Geometry check sheet. Reference: drawing and pictorial views, mm from the part's lowest x, y, z. A direction names the side the tool comes from. Coordinates: 2 decimals unless noted, no trailing zeros. Write each loop counter-clockwise with the first axis right and the second up, starting at its lowest first coordinate (ties: lowest second). Pieces come first, ordered by that corner, then holes. Notation, with made-up numbers: (-26, 18) -> (29, 18) arc R4 cw to (29, 24) -> close; hole circle Ø9 at (-16.5, -38.5). An arc over 180 degrees is marked (long way). Use a Markdown table: item, result.
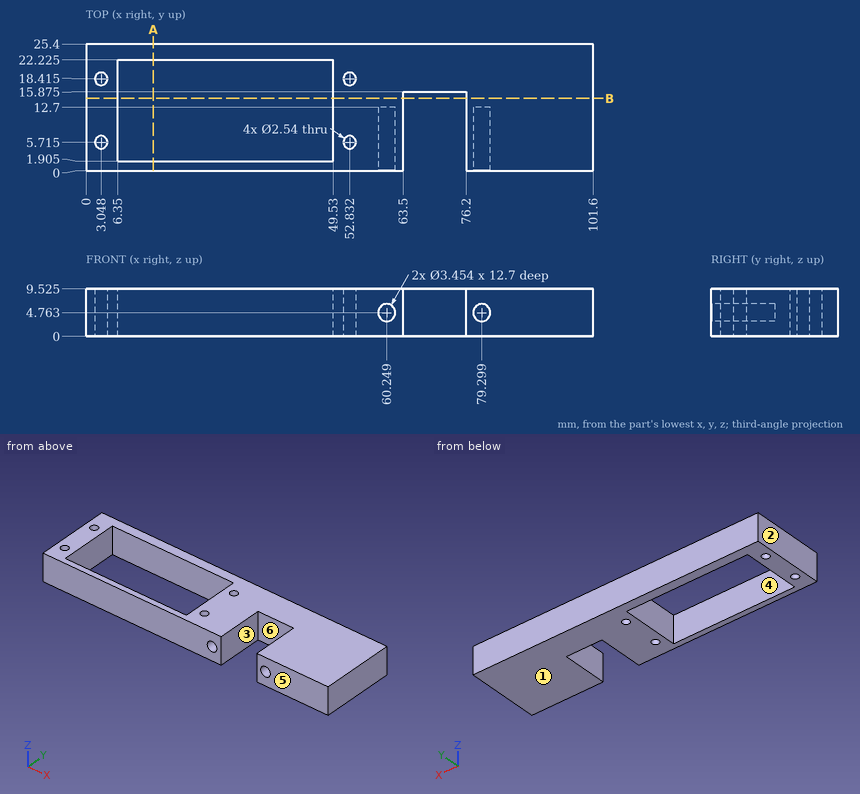
Item 1: Thickness scan on L1, parallel to Y at x = 46, z = 9.25 (1 decimal); L2, parallel to X at y = 3, z = 7.5; L3, parallel to X at y = 20.25, z = 1.75. Record the ranges inside material, lowest first. Write a range as [from, to].
Answer block:
| item | result |
|---|---|
| L1 | y = [0, 1.9], [22.2, 25.4] |
| L2 | x = [0, 6.35], [49.53, 63.5], [76.2, 101.6] |
| L3 | x = [0, 6.35], [49.53, 101.6] |
Item 2: Section check A-A on x = 13.5. Record the boundary of the cut face in (y, z) (1 decimal).
Answer block:
| item | result |
|---|---|
| outline | (0, 0) -> (1.9, 0) -> (1.9, 9.5) -> (0, 9.5) -> close; (22.2, 0) -> (25.4, 0) -> (25.4, 9.5) -> (22.2, 9.5) -> close |
Item 3: Section check B-B on y = 14.5. Count the separate pieces of the cut face and the enclosed holes in it.
Answer block:
| item | result |
|---|---|
| separate pieces | 3 |
| enclosed holes | 0 |
Item 4: Mould release check, pull along X, two halves, no side actions. Record for the marked faces 1, 2 and 3: +X half, -X half, draft (parallel to the pull), parting line (faces both ways), or undercut.
Answer block:
| item | result |
|---|---|
| face 1 | draft |
| face 2 | -X half |
| face 3 | undercut |
Item 5: Tool access check on the marked faces 4, 5 and 6. Record the directions out of +Z, -Z, +X, -X, +Y, -Y that give a thin tool (end or side, any length) a straight path to the whole face; none if there is none.
Answer block:
| item | result |
|---|---|
| face 4 | +Z, -Z |
| face 5 | +Z, -Z, +X, -X, -Y |
| face 6 | +Z, -Z, -Y |
Item 6: Depth check by flat-ended pin: P1, Ø2, axis at x = 70, z = 2, coming from the -Y side (1 decimal); P2, Ø1, axis at x = 80, z = 5.5, coming from the -Y side. Enter the tip coordinate at first touch or a pass-through.
Answer block:
| item | result |
|---|---|
| P1 | stops at y = 15.9 |
| P2 | stops at y = 12.7 |
